```python
from build123d import *

# Parameters (mm, degrees)
SKETCH1_W          = 228.6
SKETCH1_H          = 139.7
EXTRUDE1_DEPTH     = 6.35
SKETCH1_3_W        = 228.6
SKETCH1_3_H        = 139.7
SKETCH1_3_W_2      = 215.9
SKETCH1_3_H_2      = 127
EXTRUDE2_DEPTH     = 50.8
SKETCH1_6_R        = 47.625
SKETCH1_6_R_2      = 7.9375
EXTRUDE4_DEPTH     = 63.5
SKETCH16_W         = 228.6
SKETCH16_H         = 139.7
EXTRUDE3_DEPTH     = 6.35
SKETCH1_5_R        = 10.1203125
SKETCH1_5_R_2      = 7.9375
CUT_EXTRUDE2_DEPTH = 57.15


with BuildPart() as part:
    # Sketch1 → Extrude1 (new body)
    with BuildSketch(Plane.XY):
        Rectangle(SKETCH1_W, SKETCH1_H)
    extrude(amount=-EXTRUDE1_DEPTH)

    # Sketch1_3 → Extrude2 (add)
    with BuildSketch(Plane.XY):
        Rectangle(SKETCH1_3_W, SKETCH1_3_H)
        Rectangle(SKETCH1_3_W_2, SKETCH1_3_H_2, mode=Mode.SUBTRACT)
    extrude(amount=EXTRUDE2_DEPTH)

    # Sketch1_6 → Extrude4 (add)
    with BuildSketch(Plane.XY):
        with Locations(Location((0, 0, 0), (0, 0, 180))):
            Circle(SKETCH1_6_R)
        with Locations((-31.75, 0)):
            Circle(SKETCH1_6_R_2, mode=Mode.SUBTRACT)
        with Locations((31.75, 0)):
            Circle(SKETCH1_6_R_2, mode=Mode.SUBTRACT)
    extrude(amount=EXTRUDE4_DEPTH)

    # Sketch16 → Extrude3 (add)
    with BuildSketch(Plane.XY.offset(50.8)):
        Rectangle(SKETCH16_W, SKETCH16_H)
    extrude(amount=EXTRUDE3_DEPTH)

    # Sketch1_5 → Cut-Extrude2 (cut)
    with BuildSketch(Plane.XY):
        with Locations((-69.85, 0)):
            Circle(SKETCH1_5_R)
        with Locations((-31.75, 0)):
            Circle(SKETCH1_5_R_2)
        with Locations((69.85, 0)):
            Circle(SKETCH1_5_R)
        with Locations((31.75, 0)):
            Circle(SKETCH1_5_R_2)
    extrude(amount=CUT_EXTRUDE2_DEPTH, mode=Mode.SUBTRACT)


solid = part.part
```
Here's how the part is built. I have some questions about the finished solid (model axes, mm). A direction names the side the tool comes from. Coordinates: 2 decimals unless noted, no trailing zeros. Order: outer loops, then holes, each group sorted by start corner. A loop starts at its lowest first (then second) coordinate and runs counter-clockwise, first axis right, second up.
1) Imagine slicing it at B-B on x = 57. List the corners of the cut face in (y, z) for me, and give its area (3 significant figures).
2) We'd pull the mould along Y, two halves only. Please class faces 4 (the face through (59.74, 0.44, 53.93)), 5 (the face through (114.3, -1, 25)), 6 (the face through (39.1, -3, 31.3)), 7 (the face through (10.324, 46.492, 60.281)): +Y half, -Y half, draft (parallel to the pull), parting line (faces both ways), or undercut.
3) Imagine slicing it at D-D on y = 22.5. List the corners of the cut face in (x, z) for me, and give its area (3 significant figures).
4) Imagine slicing it at C-C on x = 0. List the corners of the cut face in (y, z) for me (3 decimals), and give its area (3 significant figures).
5) I need wall thicknesses on line 1 (Z direction, x = 50, y = -52.5); line 2 (Y direction, x = -69, z = 54); line 3 (Y direction, x = -31.75, z = 19). Which ranges of each line are inside material? Lowest first, please.
6) Will these pins go through, and if not, where does the flat tip stop? pin 1 (3 mm diameter, centred on x = 41, y = -43, fed in from +Z); pin 2 (14.5 mm diameter, centred on x = 31.75, y = 0, fed in from +Z).
7) Imagine slicing it at A-A on z = 31.5. State how many separate pieces and enclosed holes the cut face has, and give its area (3 significant figures).
8) Which directions (+Z, -Z, +X, -X, +Y, -Y) give clear straight access to the entire face, cutting with the end or side of a thin tool? Please do faces 1 (the face through (-49, 1, 50.8)), 2 (the face through (-32, 0, 0)), 3 (the face through (-2, 1, -6.35)).
Response values:
1. outline: (-69.85, -6.35) - (69.85, -6.35) - (69.85, 57.15) - (-69.85, 57.15) - close; hole (-63.5, 0) - (63.5, 0) - (63.5, 50.8) - (-63.5, 50.8) - close
1. area: 2,420 mm2
2. face 4: undercut
2. face 5: draft
2. face 6: undercut
2. face 7: parting line
3. outline: (-114.3, -6.35) - (114.3, -6.35) - (114.3, 57.15) - (41.97, 57.15) - (41.97, 63.5) - (-41.97, 63.5) - (-41.97, 57.15) - (-114.3, 57.15) - close; hole (-107.95, 0) - (-41.97, 0) - (-41.97, 50.8) - (-107.95, 50.8) - close; hole (41.97, 0) - (107.95, 0) - (107.95, 50.8) - (41.97, 50.8) - close
3. area: 8,350 mm2
4. outline: (-69.85, -6.35) - (69.85, -6.35) - (69.85, 57.15) - (47.625, 57.15) - (47.625, 63.5) - (-47.625, 63.5) - (-47.625, 57.15) - (-69.85, 57.15) - close; hole (-63.5, 0) - (-47.625, 0) - (-47.625, 50.8) - (-63.5, 50.8) - close; hole (47.625, 0) - (63.5, 0) - (63.5, 50.8) - (47.625, 50.8) - close
4. area: 7,860 mm2
5. line 1: z = -6.35 to 0, 50.8 to 57.15
5. line 2: y = -69.85 to -10.08, 10.08 to 69.85
5. line 3: y = -69.85 to -63.5, -35.5 to -7.94, 7.94 to 35.5, 63.5 to 69.85
6. pin 1: stops at z = 57.15
6. pin 2: stops at z = 0
7. separate pieces: 2
7. enclosed holes: 3
7. area: 11,200 mm2
8. face 1: none
8. face 2: +Z
8. face 3: -Z, +X, -X, +Y, -Y
